Print and shaded views of the part. All mm, measured from the part's lowest x, y and z. A direction names the side the tool comes from. Coordinates: 2 decimals unless noted, no trailing zeros. Order: outer loops, then holes, each group sorted by start corner. A loop starts at its lowest first (then second) coordinate and runs counter-clockwise, first axis right, second up. Notation, with made-up numbers: (-22, 23.5) -> (-7, 23.5) arc R12 ccw to (-7, 43.5) -> close; hole circle Ø6 at (-2.5, 0.25). An arc over 180 degrees is marked (long way). Write item = value, one per line. Start each with the question number.
Q1. Cut at A-A, the plane z = 59.5. List the corners of the cut face in (x, y) (1 decimal), plus the area to 3 significant figures.
Q2. Cut at B-B, the plane x = 106.5. List the corners of the cut face in (y, z).
Q3. Wall check: line 1 (X direction, y = 39, z = 18.5) (1 decimal); line 2 (Y direction, x = 45, z = 14); line 3 (Y direction, x = 98, z = 14.5) (1 decimal). Give the ranges that are in metal, low to high. Write a range as from..to.
Q4. Cut at C-C, the plane z = 49. List the corners of the cut face in (x, y) (1 decimal), plus the area to 3 significant figures.
Q5. Mould opens along Y. For the marked faces 4, 5, 6 and 7 say: +Y half, -Y half, draft (parallel to the pull), parting line (faces both ways), or undercut.
Q6. Cut at D-D, the plane x = 63.5. List the corners of the cut face in (y, z), plus the area to 3 significant figures.
Q7. 3-axis set-ups, long thin cutter, end or side, ignore diameter. For the marked faces 1, 2 and 3: which of +Z, -Z, +X, -X, +Y, -Y reach the whole face in a straight line?
Q8. Flat gauge pins, fed straight in: pin 1 (2 mm diameter, centred on x = 56.5, z = 16, fed in from +Y); pin 2 (4 mm diameter, centred on x = 76.5, z = 25, fed in from -Y); pin 3 (1 mm diameter, centred on y = 83.5, z = 62, fed in from +X). Where does each tip first touch, or does it go through?
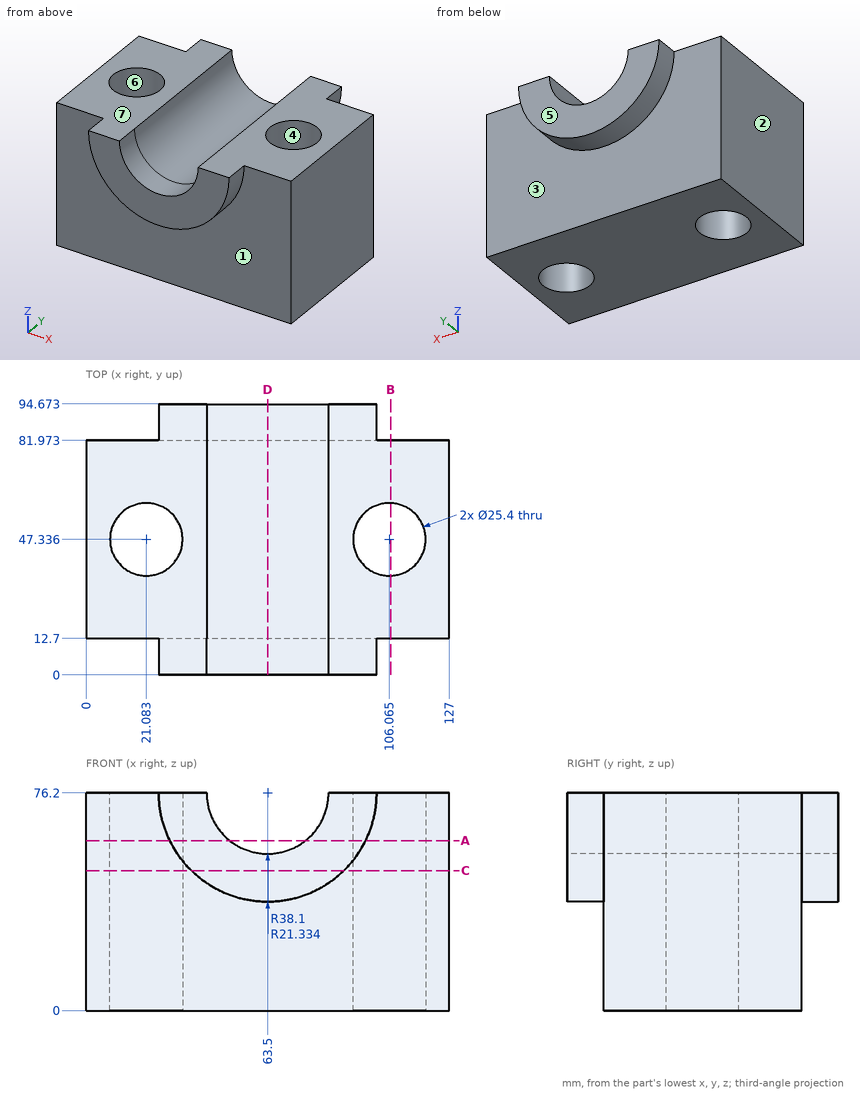
Here are the results:
q1.outline = (0, 12.7) -> (29.3, 12.7) -> (29.3, 0) -> (50.2, 0) -> (50.2, 94.7) -> (29.3, 94.7) -> (29.3, 82) -> (0, 82) -> close; (76.8, 0) -> (97.7, 0) -> (97.7, 12.7) -> (127, 12.7) -> (127, 82) -> (97.7, 82) -> (97.7, 94.7) -> (76.8, 94.7) -> close; hole circle Ø25.4 at (21.1, 47.3); hole circle Ø25.4 at (106.1, 47.3)
q1.area = 7,010 mm²
q2.outline = (12.7, 0) -> (34.64, 0) -> (34.64, 76.2) -> (12.7, 76.2) -> close; (60.03, 0) -> (81.97, 0) -> (81.97, 76.2) -> (60.03, 76.2) -> close
q3.line_1 = 0..11.5, 30.7..96.5, 115.6..127
q3.line_2 = 12.7..81.97
q3.line_3 = 12.7..37.5, 57.1..82
q4.outline = (0, 12.7) -> (36.8, 12.7) -> (36.8, 0) -> (90.2, 0) -> (90.2, 12.7) -> (127, 12.7) -> (127, 82) -> (90.2, 82) -> (90.2, 94.7) -> (36.8, 94.7) -> (36.8, 82) -> (0, 82) -> close; hole circle Ø25.4 at (21.1, 47.3); hole circle Ø25.4 at (106.1, 47.3)
q4.area = 9,140 mm²
q5.face_4 = undercut
q5.face_5 = +Y half
q5.face_6 = undercut
q5.face_7 = draft
q6.outline = (0, 38.1) -> (12.7, 38.1) -> (12.7, 0) -> (81.97, 0) -> (81.97, 38.1) -> (94.67, 38.1) -> (94.67, 54.87) -> (0, 54.87) -> close
q6.area = 4,230 mm²
q7.face_1 = -Z, -Y
q7.face_2 = +Z, -Z, -X, +Y, -Y
q7.face_3 = -Z, +Y
q8.pin_1 = 81.97
q8.pin_2 = 12.7
q8.pin_3 = 99.05
